from build123d import *

# Parameters (mm, degrees)
SKETCH1_W           = 90
SKETCH1_H           = 90
BOSS_EXTRUDE1_DEPTH = 19
SKETCH9_W           = 44
SKETCH9_H           = 19
BOSS_EXTRUDE2_DEPTH = 65
SKETCH2_R           = 28.5
CUT_EXTRUDE1_DEPTH  = 3
SKETCH4_W           = 23
SKETCH4_H           = 23
CUT_EXTRUDE3_DEPTH  = 20
SKETCH11_R          = 2.5
CUT_EXTRUDE4_DEPTH  = 10
SKETCH12_R          = 2.5
CUT_EXTRUDE5_DEPTH  = 10


with BuildPart() as part:
    # Sketch1 → Boss-Extrude1 (new body)
    with BuildSketch(Plane(origin=(0, 0, 0), x_dir=(1, 0, 0), z_dir=(0, 1, 0))):
        with Locations((45, 45)):
            Rectangle(SKETCH1_W, SKETCH1_H)
    extrude(amount=BOSS_EXTRUDE1_DEPTH)

    # Sketch9 → Boss-Extrude2 (add, symmetric)
    with BuildSketch(Plane(origin=(45, 0, 0), x_dir=(0, 0, -1), z_dir=(1, 0, 0))):
        with Locations((45, 9.5)):
            Rectangle(SKETCH9_W, SKETCH9_H)
    extrude(amount=BOSS_EXTRUDE2_DEPTH, both=True)

    # Sketch2 → Cut-Extrude1 (cut)
    with BuildSketch(Plane(origin=(0, 19, 0), x_dir=(1, 0, 0), z_dir=(0, 1, 0))):
        with Locations((45, 45)):
            Circle(SKETCH2_R)
    extrude(amount=-CUT_EXTRUDE1_DEPTH, mode=Mode.SUBTRACT)

    # Sketch4 → Cut-Extrude3 (cut, through all)
    with BuildSketch(Plane(origin=(0, 19, 0), x_dir=(1, 0, 0), z_dir=(0, 1, 0))):
        with Locations((11.5, 11.5)):
            Rectangle(SKETCH4_W, SKETCH4_H)
        with Locations((11.5, 78.5)):
            Rectangle(SKETCH4_W, SKETCH4_H)
        with Locations((78.5, 78.5)):
            Rectangle(SKETCH4_W, SKETCH4_H)
        with Locations((78.5, 11.5)):
            Rectangle(SKETCH4_W, SKETCH4_H)
    extrude(amount=-CUT_EXTRUDE3_DEPTH, mode=Mode.SUBTRACT)

    # Sketch11 → Cut-Extrude4 (cut)
    with BuildSketch(Plane(origin=(110, 0, 0), x_dir=(0, 0, -1), z_dir=(1, 0, 0))):
        with Locations((45, 9.5)):
            Circle(SKETCH11_R)
    extrude(amount=-CUT_EXTRUDE4_DEPTH, mode=Mode.SUBTRACT)

    # Sketch12 → Cut-Extrude5 (cut)
    with BuildSketch(Plane.ZY.offset(20)):
        with Locations((-45, 9.5)):
            Circle(SKETCH12_R)
    extrude(amount=-CUT_EXTRUDE5_DEPTH, mode=Mode.SUBTRACT)


solid = part.part
Geometry: final body of the model. Coordinates: model frame, mm. A direction names the side the tool comes from. Coordinates: 2 decimals unless noted, no trailing zeros. Write each loop counter-clockwise with the first axis right and the second up, starting at its lowest first coordinate (ties: lowest second). Pieces come first, ordered by that corner, then holes. Notation, with made-up numbers: (36.25, -26.5) - (84.25, -26.5) arc R30 cw to (84.25, -2.5) - close; hole circle Ø4 at (42.25, 9). An arc over 180 degrees is marked (long way). Return JSON: item names as keys, results as strings.
Item 1: Section query B-B (y = 9.5). Output: boundary loops of the cut face in (x, z).
Completed:
{"outline": "(-20, -67) - (23, -67) - (23, -90) - (67, -90) - (67, -67) - (110, -67) - (110, -47.5) - (100, -47.5) - (100, -42.5) - (110, -42.5) - (110, -23) - (67, -23) - (67, 0) - (23, 0) - (23, -23) - (-20, -23) - (-20, -42.5) - (-10, -42.5) - (-10, -47.5) - (-20, -47.5) - close"}
Item 2: Reachability of faces 4 (the face through (23, 10, -11)), 5 (the face through (67, 10, -11)), 6 (the face through (89, 9, -67)) from +Z, -Z, +X, -X, +Y, -Y: full face, straight path, thin tool, end or side. Return the list, or none.
Completed:
{"face 4": "+Z, -X, +Y, -Y", "face 5": "+Z, +X, +Y, -Y", "face 6": "-Z, +X, +Y, -Y"}
Item 3: Pin query (flat end, axial travel): pin 1 Ø3 at (y, z) = (7, -18.5) entering from -X; pin 2 Ø9.5 at (x, y) = (-5.5, 6.5) entering from +Z; pin 3 Ø1.5 at (y, z) = (9, -45.5) entering from -X. Return the tip coordinate at first contact, or that it passes through.
Completed:
{"pin 1": "stops at x = 23", "pin 2": "stops at z = -23", "pin 3": "stops at x = -10"}
Item 4: Section query A-A (x = 45). Output: boundary loops of the cut face in (y, z), and give its area (3 significant figures).
Completed:
{"outline": "(0, -90) - (19, -90) - (19, -73.5) - (16, -73.5) - (16, -16.5) - (19, -16.5) - (19, 0) - (0, 0) - close", "area": "1,540 mm2"}
Item 5: Line query: L1, parallel to X at y = 17.7, z = -45; L2, parallel to Y at x = 103.25, z = -45; L3, parallel to Z at x = 45, y = 18.15. Output: solid intervals per line, ascending.
Completed:
{"L1": "x = -20 to 16.5, 73.5 to 110", "L2": "y = 0 to 7, 12 to 19", "L3": "z = -90 to -73.5, -16.5 to 0"}
Item 6: Section query D-D (y = 3). Output: boundary loops of the cut face in (x, z), and give its area (3 significant figures).
Completed:
{"outline": "(-20, -67) - (23, -67) - (23, -90) - (67, -90) - (67, -67) - (110, -67) - (110, -23) - (67, -23) - (67, 0) - (23, 0) - (23, -23) - (-20, -23) - close", "area": "7,740 mm2"}
Item 7: Section query C-C (z = -45). Output: boundary loops of the cut face in (x, y), and give its area (3 significant figures).
Completed:
{"outline": "(-20, 0) - (110, 0) - (110, 7) - (100, 7) - (100, 12) - (110, 12) - (110, 19) - (73.5, 19) - (73.5, 16) - (16.5, 16) - (16.5, 19) - (-20, 19) - (-20, 12) - (-10, 12) - (-10, 7) - (-20, 7) - close", "area": "2,200 mm2"}
Item 8: Pull-direction query (X, two-part tool) for faces 1 (the face through (45, 16, -45)), 2 (the face through (67, 10, -78)), 3 (the face through (2, 9, -23)); classes: +X half, -X half, draft (parallel to the pull), parting line (faces both ways), or undercut.
Completed:
{"face 1": "undercut", "face 2": "+X half", "face 3": "draft"}
